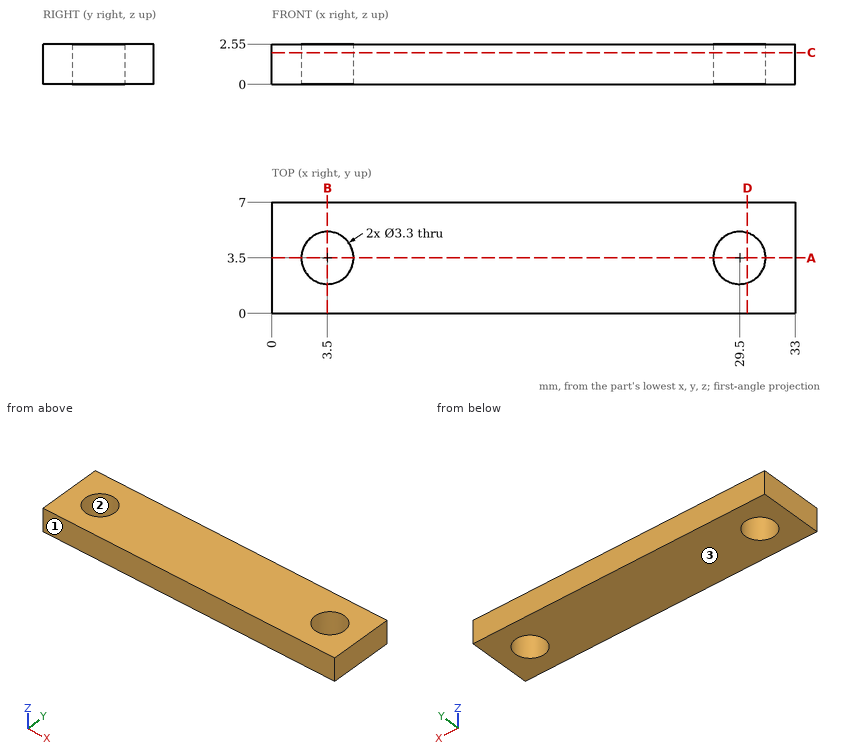
The figure shows three views and two pictorial views of one solid part (mm, origin at its lowest corner). Answer the questions. Round coordinates to 2 decimals unless told otherwise and drop trailing zeros. Write each loop counter-clockwise with the first axis right and the second up, starting at its lowest first coordinate (ties: lowest second). Pieces come first, ordered by that corner, then holes. Notation, with made-up numbers: (11.25, -33.75) - (44.25, -33.75) arc R18 cw to (44.25, -13.75) - close; hole circle Ø9 at (32, 0.5). An arc over 180 degrees is marked (long way). Answer in a Markdown table with one row per item. Add a question column.
1. A cutting plane is placed at A-A, the plane y = 3.5. Determine the outline of the cut face in (x, z), and give its area (3 significant figures).
2. Find the intervals of material crossed by line 1 along Y through (x, z) = (3.5, 0.75); line 2 along X through (y, z) = (2.25, 1.3); line 3 along X through (y, z) = (2, 0.5), in increasing order. Write a range as from..to.
3. A cutting plane is placed at B-B, the plane x = 3.5. Determine the outline of the cut face in (y, z).
4. The mould has two halves that part along Y. Classify the marked faces 1, 2 and 3: +Y half, -Y half, draft (parallel to the pull), parting line (faces both ways), or undercut.
5. A cutting plane is placed at C-C, the plane z = 2. Determine the outline of the cut face in (x, y), and give its area (3 significant figures).
6. A cutting plane is placed at D-D, the plane x = 30. Determine the outline of the cut face in (y, z), and give its area (3 significant figures).
Worked out:
| question | item | result |
|---|---|---|
| 1 | outline | (0, 0) - (1.85, 0) - (1.85, 2.55) - (0, 2.55) - close; (5.15, 0) - (27.85, 0) - (27.85, 2.55) - (5.15, 2.55) - close; (31.15, 0) - (33, 0) - (33, 2.55) - (31.15, 2.55) - close |
| 1 | area | 67.3 mm^2 |
| 2 | line 1 | 0..1.85, 5.15..7 |
| 2 | line 2 | 0..2.42, 4.58..28.42, 30.58..33 |
| 2 | line 3 | 0..2.81, 4.19..28.81, 30.19..33 |
| 3 | outline | (0, 0) - (1.85, 0) - (1.85, 2.55) - (0, 2.55) - close; (5.15, 0) - (7, 0) - (7, 2.55) - (5.15, 2.55) - close |
| 4 | face 1 | -Y half |
| 4 | face 2 | undercut |
| 4 | face 3 | draft |
| 5 | outline | (0, 0) - (33, 0) - (33, 7) - (0, 7) - close; hole circle Ø3.3 at (3.5, 3.5); hole circle Ø3.3 at (29.5, 3.5) |
| 5 | area | 214 mm^2 |
| 6 | outline | (0, 0) - (1.93, 0) - (1.93, 2.55) - (0, 2.55) - close; (5.07, 0) - (7, 0) - (7, 2.55) - (5.07, 2.55) - close |
| 6 | area | 9.83 mm^2 |
